Work out the finished part from the listing and answer in its coordinate system (mm). A direction names the side the tool comes from. Coordinates: 2 decimals unless noted, no trailing zeros. Order: outer loops, then holes, each group sorted by start corner. A loop starts at its lowest first (then second) coordinate and runs counter-clockwise, first axis right, second up. Notation, with made-up numbers: M 3,69 L 42,69 A18 ccw 42,80 Z; hole C 25,17.5 d5. An arc over 180 degrees is marked long. Answer in a Markdown table with one row per item. Add a question column.
Item 1: The part is cut by section A-A (z = 0). Write down the section's boundary in (x, y), then the cut area to 3 significant figures.
Item 2: The mould has two halves that part along X. Classify faces 4 (the face through (0, 3, 39.688)), 5 (the face through (13, 3, -30.362)): released by +X, released by -X, zero draft, split by the parting line, or undercut.
Item 3: Flat-ended cylindrical pins translate along their axes: pin 1 Ø1.5 at (x, y) = (-31.5, 1.5) entering from -Z; pin 2 Ø1.8 at (x, y) = (-11.5, 4) entering from +Z; pin 3 Ø3 at (y, z) = (3, 37.5) entering from +X. Find the tip coordinate at first contact, or state that the pin passes through.
Item 4: Consider line 1 (X direction, y = 4.25, z = 0.5); line 2 (X direction, y = 6, z = -27); line 3 (X direction, y = 4, z = -30). Determine where each line is inside the solid, lowest interval first. Write a range as from..to.
Item 5: The part is cut by section D-D (x = 30). Write down the section's boundary in (y, z).
Item 6: The part is cut by section B-B (x = 0). Write down the section's boundary in (y, z), then the cut area to 3 significant figures.
Item 7: Which of the six approach directions +Z, -Z, +X, -X, +Y, -Y give full straight-line access (tool end or side, diameter ignored) to faces 1 (the face through (12.106, 3, -29)), 2 (the face through (-21, 3, -33.538)), 3 (the face through (-14.146, 3, 32))?
Item 8: The part is cut by section C-C (z = 31.5). Write down the section's boundary in (x, y), then the cut area to 3 significant figures.
from build123d import *

# Parameters (mm, degrees)
SKETCH1_R           = 2.15265
SKETCH1_R_2         = 8.73125
BOSS_EXTRUDE1_DEPTH = 6.35
CUT_EXTRUDE1_DEPTH  = 57.484668827


with BuildPart() as part:
    # Sketch1 → Boss-Extrude1 (new body)
    with BuildSketch(Plane(origin=(0, 0, 0), x_dir=(1, 0, 0), z_dir=(0, 1, 0))):
        Polygon((23.8125, 39.6875), (-23.8125, 39.6875), (-39.6875, 23.8125), (-39.6875, -23.8125), (-23.8125, -39.6875), (23.8125, -39.6875), (39.6875, -23.8125), (39.6875, 23.8125), align=None)
        with Locations(Location((-13.748153285, -7.9375, 0), (0, 0, 270))):
            Circle(SKETCH1_R, mode=Mode.SUBTRACT)
        with Locations(Location((13.748153285, -7.9375, 0), (0, 0, 270))):
            Circle(SKETCH1_R, mode=Mode.SUBTRACT)
        with Locations(Location((0, 0, 0), (0, 0, 270))):
            Circle(SKETCH1_R_2, mode=Mode.SUBTRACT)
        with Locations(Location((0, 15.875, 0), (0, 0, 270))):
            Circle(SKETCH1_R, mode=Mode.SUBTRACT)
    extrude(amount=BOSS_EXTRUDE1_DEPTH)

    # Sketch2 → Cut-Extrude1 (cut, through all)
    with BuildSketch(Plane(origin=(0, 6.35, 0), x_dir=(1, 0, 0), z_dir=(0, 1, 0))):
        Polygon((-8.0375, 39.6875), (-23.7125, 39.6875), (-23.7125, 33.5375), (-17.8038, 33.5375), (-17.8038, 30.3625), (-19.84375, 30.3625), (-19.84375, 27.3875), (-17.8038, 27.3875), (-17.8038, 26.59375), (-14.3462, 26.59375), (-14.3462, 27.3875), (-12.10625, 27.3875), (-12.10625, 30.3625), (-14.1462, 30.3625), (-14.1462, 33.5375), (-8.0375, 33.5375), align=None)
        Polygon((23.7125, 39.6875), (8.0375, 39.6875), (8.0375, 33.5375), (14.1462, 33.5375), (14.1462, 30.3625), (12.10625, 30.3625), (12.10625, 27.3875), (14.3462, 27.3875), (14.3462, 26.59375), (17.8038, 26.59375), (17.8038, 27.3875), (19.84375, 27.3875), (19.84375, 30.3625), (17.8038, 30.3625), (17.8038, 33.5375), (23.7125, 33.5375), align=None)
        Polygon((-23.7125, -33.5375), (-23.7125, -39.6875), (-8.0375, -39.6875), (-8.0375, -33.5375), (-14.1462, -33.5375), (-14.1462, -30.3625), (-12.10625, -30.3625), (-12.10625, -27.3875), (-14.3462, -27.3875), (-14.3462, -26.59375), (-17.8038, -26.59375), (-17.8038, -27.3875), (-19.84375, -27.3875), (-19.84375, -30.3625), (-17.8038, -30.3625), (-17.8038, -33.5375), align=None)
        Polygon((8.0375, -33.5375), (8.0375, -39.6875), (23.7125, -39.6875), (23.7125, -33.5375), (17.8038, -33.5375), (17.8038, -30.3625), (19.84375, -30.3625), (19.84375, -27.3875), (17.8038, -27.3875), (17.8038, -26.59375), (14.3462, -26.59375), (14.3462, -27.3875), (12.10625, -27.3875), (12.10625, -30.3625), (14.1462, -30.3625), (14.1462, -33.5375), align=None)
    extrude(amount=-CUT_EXTRUDE1_DEPTH, mode=Mode.SUBTRACT)


solid = part.part
Reply:
| question | item | result |
|---|---|---|
| 1 | outline | M -39.69,0 L -8.73,0 L -8.73,6.35 L -39.69,6.35 Z; M 8.73,0 L 39.69,0 L 39.69,6.35 L 8.73,6.35 Z |
| 1 | area | 393 mm2 |
| 2 | face 4 | zero draft |
| 2 | face 5 | undercut |
| 3 | pin 1 | stops at z = -32.75 |
| 3 | pin 2 | stops at z = 33.54 |
| 3 | pin 3 | stops at x = 27.5 |
| 4 | line 1 | x = -39.69..-8.72, 8.72..39.69 |
| 4 | line 2 | x = -36.5..-17.8, -14.35..14.35, 17.8..36.5 |
| 4 | line 3 | x = -33.5..-19.84, -12.11..12.11, 19.84..33.5 |
| 5 | outline | M 0,-33.5 L 6.35,-33.5 L 6.35,33.5 L 0,33.5 Z |
| 6 | outline | M 0,-39.69 L 6.35,-39.69 L 6.35,-18.03 L 0,-18.03 Z; M 0,-13.72 L 6.35,-13.72 L 6.35,-8.73 L 0,-8.73 Z; M 0,8.73 L 6.35,8.73 L 6.35,39.69 L 0,39.69 Z |
| 6 | area | 366 mm2 |
| 7 | face 1 | +Y, -Y |
| 7 | face 2 | -Z, +Y, -Y |
| 7 | face 3 | +Z, +Y, -Y |
| 8 | outline | M -32,0 L -17.8,0 L -17.8,6.35 L -32,6.35 Z; M -14.15,0 L 14.15,0 L 14.15,6.35 L -14.15,6.35 Z; M 17.8,0 L 32,0 L 32,6.35 L 17.8,6.35 Z |
| 8 | area | 360 mm2 |
